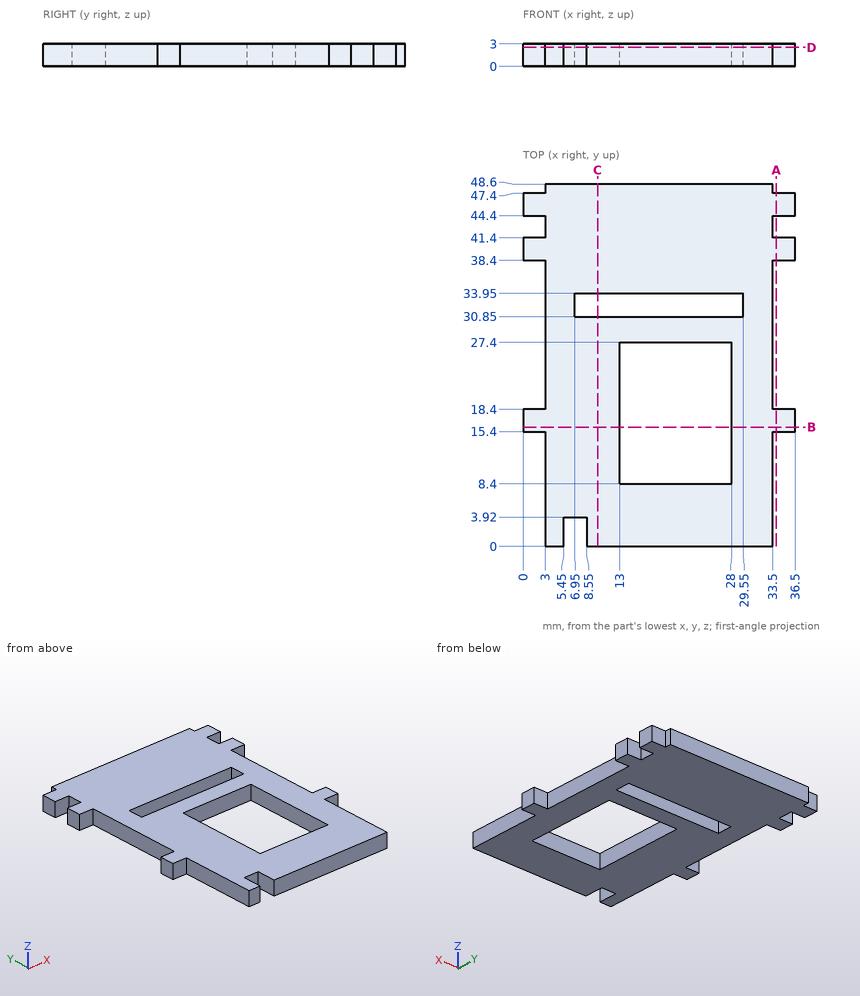
Geometry: see drawing. Coordinates: mm, zero at the bounding-box minimum. Give positions to 0.01 mm unless a question says otherwise; leave off trailing zeros. Order: outer loops, then holes, each group sorted by start corner. A loop starts at its lowest first (then second) coordinate and runs counter-clockwise, first axis right, second up. Notation, with made-up numbers: M -40,36.25 L -26,36.25 A11 ccw -26,56.25 Z; hole C 65.5,83 d2. An arc over 180 degrees is marked long. Answer as CSV lines item,"result". Start each with the question number.
1) Cut plane B-B (y = 16). Output: boundary loops of the cut face in (x, z), then the cut area to 3 significant figures.
2) Cut plane A-A (x = 34). Output: boundary loops of the cut face in (y, z).
3) Line query: line 1 (Y direction, x = 22.5, z = 2.9); line 2 (Y direction, x = 11, z = 1.75); line 3 (Y direction, x = 34, z = 1.65). Output: solid intervals per line, ascending. Write a range as from..to.
4) Cut plane D-D (z = 2.55). State how many separate pieces and enclosed holes the cut face has, then the cut area to 3 significant figures.
5) First-contact query: P1, Ø1.5, axis at y = 20, z = 1.5, coming from the +X side; P2, Ø1.5, axis at x = 1.5, z = 1, coming from the -Y side; P3, Ø1.5, axis at y = 32, z = 1.5, coming from the -X side. Flat tips, straight axial feed; report the tip coordinate or a pass-through.
6) Cut plane C-C (x = 10). Output: boundary loops of the cut face in (y, z), then the cut area to 4 significant figures.
Findings below:
1,outline,"M 0,0 L 13,0 L 13,3 L 0,3 Z; M 28,0 L 36.5,0 L 36.5,3 L 28,3 Z"
1,area,"64.5 mm²"
2,outline,"M 15.4,0 L 18.4,0 L 18.4,3 L 15.4,3 Z; M 38.4,0 L 41.4,0 L 41.4,3 L 38.4,3 Z; M 44.4,0 L 47.4,0 L 47.4,3 L 44.4,3 Z"
3,line 1,"y = 0..8.4, 27.4..30.85, 33.95..48.6"
3,line 2,"y = 0..30.85, 33.95..48.6"
3,line 3,"y = 15.4..18.4, 38.4..41.4, 44.4..47.4"
4,separate pieces,"1"
4,enclosed holes,"2"
4,area,"1,170 mm²"
5,P1,"stops at x = 33.5"
5,P2,"stops at y = 15.4"
5,P3,"stops at x = 3"
6,outline,"M 0,0 L 30.85,0 L 30.85,3 L 0,3 Z; M 33.95,0 L 48.6,0 L 48.6,3 L 33.95,3 Z"
6,area,"136.5 mm²"
